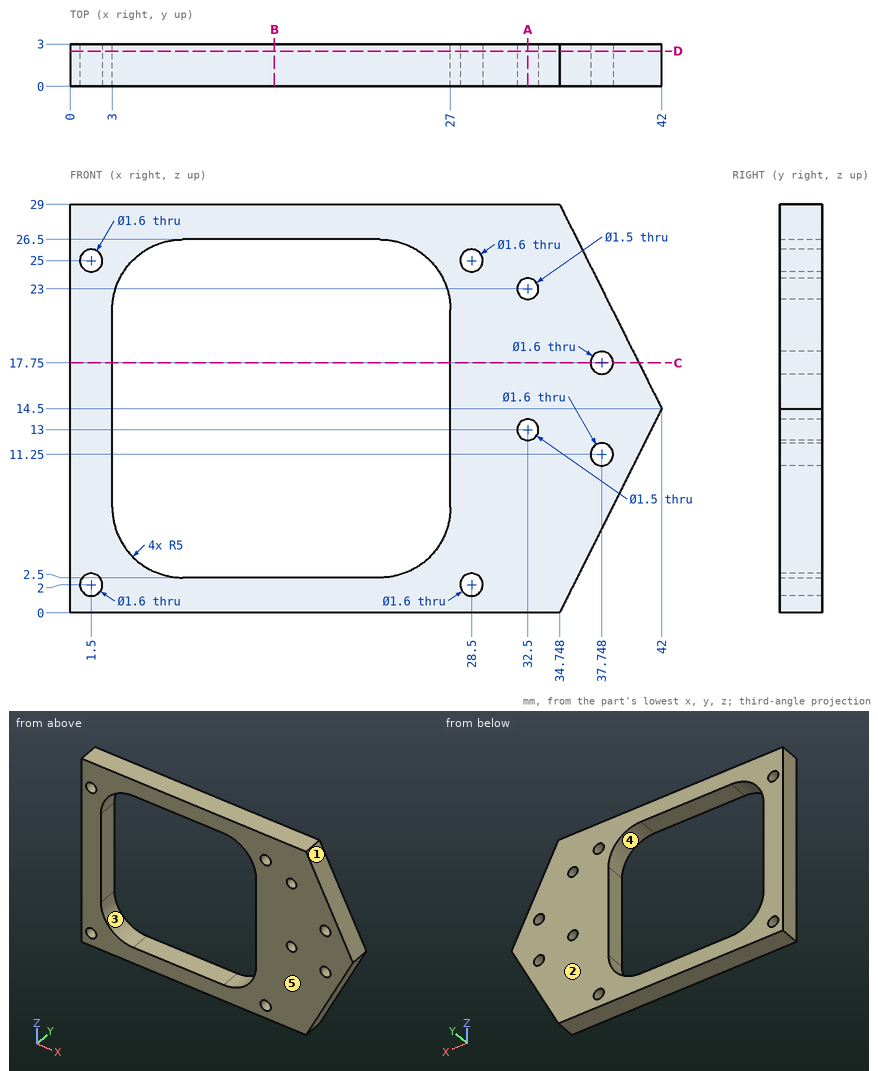
Could you check a few things on this drawing? It's one solid part, dimensions in mm from its lowest x, y, z. A direction names the side the tool comes from. Round coordinates to 2 decimals unless told otherwise and drop trailing zeros. Write each loop counter-clockwise with the first axis right and the second up, starting at its lowest first coordinate (ties: lowest second). Pieces come first, ordered by that corner, then holes. Notation, with made-up numbers: M 72.5,-25.5 L 84.5,-25.5 A16 ccw 84.5,-7.5 Z; hole C -6,-27.75 d3. An arc over 180 degrees is marked long. Answer as CSV lines item,"result". Start each with the question number.
1. I need wall thicknesses on probe 1 along Z at (x, y) = (15, 0.9); probe 2 along Z at (x, y) = (32, 0.5); probe 3 along X at (y, z) = (1.85, 13). Which ranges of each line are inside material? Lowest first, please.
2. Suppose I cut it at D-D on y = 2.5. Count the separate pieces of the cut face and the enclosed holes in it.
3. Suppose I cut it at B-B on x = 14.5. Write out the boundary of the cut face in (y, z), then the cut area to 3 significant figures.
4. Suppose I cut it at C-C on z = 17.75. Write out the boundary of the cut face in (x, y) (1 decimal).
5. On a 3-axis mill with a long thin cutter (end or side, diameter ignored), from which of +Z, -Z, +X, -X, +Y, -Y can I reach the whole of each face in a straight line? I mean the marked faces 4 and 5. Say none if no direction works.
6. Thinking about a two-plate mould opening in X: for the marked faces 1, 2 and 3, which applies, released by +X, released by -X, zero draft, split by the parting line, or undercut?
7. Suppose I cut it at A-A on x = 32.5. Write out the boundary of the cut face in (y, z).
Check result:
1,probe 1,"z = 0 to 2.5, 26.5 to 29"
1,probe 2,"z = 0 to 12.44, 13.56 to 22.44, 23.56 to 29"
1,probe 3,"x = 0 to 3, 27 to 31.75, 33.25 to 41.25"
2,separate pieces,"1"
2,enclosed holes,"9"
3,outline,"M 0,0 L 3,0 L 3,2.5 L 0,2.5 Z; M 0,26.5 L 3,26.5 L 3,29 L 0,29 Z"
3,area,"15.0 mm2"
4,outline,"M 0,0 L 3,0 L 3,3 L 0,3 Z; M 27,0 L 36.9,0 L 36.9,3 L 27,3 Z; M 38.5,0 L 40.4,0 L 40.4,3 L 38.5,3 Z"
5,face 4,"+Y, -Y"
5,face 5,"+Z, -Z, +X, -X, -Y"
6,face 1,"released by +X"
6,face 2,"zero draft"
6,face 3,"undercut"
7,outline,"M 0,0 L 3,0 L 3,12.25 L 0,12.25 Z; M 0,13.75 L 3,13.75 L 3,22.25 L 0,22.25 Z; M 0,23.75 L 3,23.75 L 3,29 L 0,29 Z"
